from build123d import *

# Parameters (mm, degrees)
F0_R     = 4.7625
F1_DEPTH = 12.7
F3_DEPTH = 12.701
F4_R     = 1.5875
F5_R     = 2.38125
F5_R_2   = 2.4756195987
F6_DEPTH = 101.6
F7_R     = 4.7625
F8_DEPTH = 4.7625
F9_DEPTH = 36.322
F10_R    = 2.032


with BuildPart() as f1:
    # F0 (on Front) → F1 (new body)
    with BuildSketch(Plane.XZ):
        with BuildLine():
            Line((0, -8.3197675008), (-20.6375, -8.3197675008))
            ThreePointArc((-20.6375, -8.3197675008), (-31.75, -19.4322675008), (-20.6375, -30.5447675008))
            Line((-20.6375, -30.5447675008), (4.7625, -30.5447675008))
            Line((4.7625, -30.5447675008), (53.975, -30.5447675008))
            Line((53.975, -30.5447675008), (53.975, -21.0070675008))
            Line((53.975, -21.0070675008), (0, -21.0070675008))
            Line((0, -21.0070675008), (0, -8.3197675008))
        make_face()
        with Locations((-20.6375, -19.4322675008)):
            Circle(F0_R, mode=Mode.SUBTRACT)
    extrude(amount=F1_DEPTH)

    # F2 (on Front) → F3 (cut, through all)
    with BuildSketch(Plane.XZ):
        Polygon((-19.3086979003, -7.7764257723), (-22.3058979003, -7.62272316), (-22.3058979003, -16.6143205299), (-19.3086979003, -16.6143205299), align=None)
    extrude(amount=F3_DEPTH, mode=Mode.SUBTRACT)

    # F4
    f4_edges = [f1.edges().sort_by_distance(p)[0] for p in [
        (-19.308698, -6.35, -8.319768),
        (-22.305898, -6.35, -8.445726),
        (-22.305898, -12.7, -11.708646),
        (-19.308698, -12.7, -11.589334),
        (-20.458601, -12.7, -24.191406),
        (-19.308698, 0, -11.589334),
        (-22.305898, 0, -11.708646),
        (-20.458601, 0, -24.191406),
    ]]
    fillet(f4_edges, radius=F4_R)

    # F5 (on Top) → F6 (cut)
    with BuildSketch(Plane.XY):
        with Locations((46.0375, -6.5245353617)):
            Circle(F5_R)
        with Locations((15.875, -6.5245353617)):
            Circle(F5_R_2)
    extrude(amount=F6_DEPTH, mode=Mode.SUBTRACT)

    # F7 (on face) → F8 (cut)
    with BuildSketch(Plane.XY.offset(-21.0070675008)):
        with Locations((15.875, -6.5245353617)):
            Circle(F7_R)
        with Locations((46.0375, -6.5245353617)):
            Circle(F7_R)
    extrude(amount=-F8_DEPTH, mode=Mode.SUBTRACT)

    # F5 (on Top) → F9 (cut)
    with BuildSketch(Plane.XY):
        with Locations((15.875, -6.5245353617)):
            Circle(F5_R_2)
        with Locations((46.0375, -6.5245353617)):
            Circle(F5_R)
    extrude(amount=-F9_DEPTH, mode=Mode.SUBTRACT)

    # F10
    f10_edges = [f1.edges().sort_by_distance(p)[0] for p in [
        (0, -6.35, -8.319768),
        (0, -6.35, -21.007068),
    ]]
    fillet(f10_edges, radius=F10_R)


solid = f1.part
Check sheet for the modelled part. Datum: model origin and axes. Units: mm. A direction names the side the tool comes from. Round coordinates to 2 decimals unless told otherwise and drop trailing zeros. Loops run counter-clockwise (first coordinate to the right, second up) from the corner with the lowest first, then second, coordinate; pieces in that order, holes last. Notation, with made-up numbers: M 42.5,73 L 76.5,73 A10 cw 76.5,89 Z; hole C -29.75,19 d8. An arc over 180 degrees is marked long. One line per item, written item: value.
(1) Sectioned sample at A-A, the plane z = -13. Record the cut outline in (x, y) (1 decimal).
Computed values:
outline: M -29.7,-12.7 L -23.9,-12.7 A1.6 ccw -22.3,-11.1 L -22.3,-1.6 A1.6 ccw -23.9,0 L -29.7,0 Z; M -19.3,-11.1 A1.6 ccw -17.7,-12.7 L 0,-12.7 L 0,0 L -17.7,0 A1.6 ccw -19.3,-1.6 Z
(2) Sectioned sample at B-B, the plane x = 17.5. Record the cut outline in (y, z).
Computed values:
outline: M -12.7,-30.54 L -8.39,-30.54 L -8.39,-25.77 L -11,-25.77 L -11,-21.01 L -12.7,-21.01 Z; M -4.66,-30.54 L 0,-30.54 L 0,-21.01 L -2.05,-21.01 L -2.05,-25.77 L -4.66,-25.77 Z
(3) Thickness scan on line 1 (X direction, y = -5.75, z = -22.25) (3 decimals); line 2 (X direction, y = -3.5, z = -23.5) (3 decimals); line 3 (X direction, y = -5.25, z = -28.5) (3 decimals). Record the ranges inside material, lowest first.
Computed values:
line 1: x = -31.387 to -24.477, -16.798 to 11.176, 20.574 to 41.338, 50.737 to 53.975
line 2: x = -30.979 to -23.114, -18.161 to 12.196, 19.554 to 42.359, 49.716 to 53.975
line 3: x = -27.061 to 13.753, 17.997 to 44.026, 48.049 to 53.975
(4) Sectioned sample at C-C, the plane y = -3. Record the cut outline in (x, z) (1 decimal), then the cut area to 3 significant figures.
Computed values:
outline: M -24.4,-9 A11.1 ccw -20.6,-30.5 L 54,-30.5 L 54,-21 L 49.2,-21 L 49.2,-25.8 L 42.8,-25.8 L 42.8,-21 L 19.1,-21 L 19.1,-25.8 L 12.7,-25.8 L 12.7,-21 L 2,-21 A2 cw 0,-19 L 0,-10.4 A2 ccw -2,-8.3 L -17.7,-8.3 A1.6 ccw -19.3,-9.9 L -19.3,-14.9 A4.8 cw long -22.3,-15 L -22.3,-10.5 A1.6 ccw Z
area: 1,010 mm^2
(5) Release check for a two-part mould opening along X. For faces 1 (the face through (-31.617, -6.261, -21.147)), 2 (the face through (18, -9, -25.77)), 3 (the face through (0.579, -6.439, -20.396)) record: +X half, -X half, draft (parallel to the pull), parting line (faces both ways), or undercut.
Computed values:
face 1: -X half
face 2: undercut
face 3: +X half
(6) Sectioned sample at D-D, the plane x = 31. Record the cut outline in (y, z), then the cut area to 3 significant figures.
Computed values:
outline: M -12.7,-30.54 L 0,-30.54 L 0,-21.01 L -12.7,-21.01 Z
area: 121 mm^2
(7) Depth check by flat-ended pin: pin 1 Ø7.5 at (x, y) = (46.04, -6.52) entering from +Z; pin 2 Ø4 at (x, y) = (15.88, -6.52) entering from -Z; pin 3 Ø1 at (x, y) = (33, -5.5) entering from +Z; pin 4 Ø3.5 at (y, z) = (-8, -12.5) entering from +X. Enter the tip coordinate at first touch or a pass-through.
Computed values:
pin 1: stops at z = -25.77
pin 2: passes through
pin 3: stops at z = -21.01
pin 4: stops at x = 0
(8) Access from +Z, -Z, +X, -X, +Y, -Y to the whole of each face (thin tool, end or side, straight path). Record for faces 4 (the face through (-22.759, -0.477, -11.975)), 5 (the face through (-22.306, -6, -13)), 6 (the face through (0, -6, -15)), 7 (the face through (11.117, -6.315, -23.355)).
Computed values:
face 4: +Z, +Y
face 5: +Z, +Y, -Y
face 6: +Z, +X, +Y, -Y
face 7: +Z
